Autodesk Fusion 360 part; units mm, degrees
sketch "Sketch1" plane through (0, 0, 0) normal (0, 0, 1) x (1, 0, 0)
  circle A0 centre (0, 0) radius 12.07
  circle A1 centre (0, 0) radius 3.2
  dimension "d1" = 24.14
  dimension "d2" = 6.4
extrude "Extrude1" add sketch "Sketch1" against normal blind 12.4 contours A0 | A1
extrude "Extrude2" add sketch "Sketch1" along normal blind 1 contours A1
sketch "Sketch2" plane through (0, 0, 1) normal (0, 0, 1) x (-1, 0, 0)
  circle A0 centre (0, 0) radius 3.2
  circle A1 centre (0, 0) radius 1
  dimension "d7" = 2
extrude "Extrude3" add sketch "Sketch2" along normal blind 4.7 contours A1
sketch "Sketch3" plane through (0, 0, 0) normal (0, 0, 1) x (1, 0, 0)
  line L0 (0, 0) -> (-8.25, 0) construction
  circle A0 centre (-8.25, 0) radius 0.75
  circle A1 centre (-4.125, -7.1447) radius 0.75
  circle A2 centre (4.125, -7.1447) radius 0.75
  circle A3 centre (8.25, 0) radius 0.75
  circle A4 centre (4.125, 7.1447) radius 0.75
  circle A5 centre (-4.125, 7.1447) radius 0.75
  dimension "d10" = 8.25
  dimension "d11" = 1.5
  dimension "d13" = 360
extrude "Extrude4" cut sketch "Sketch3" against normal blind 2
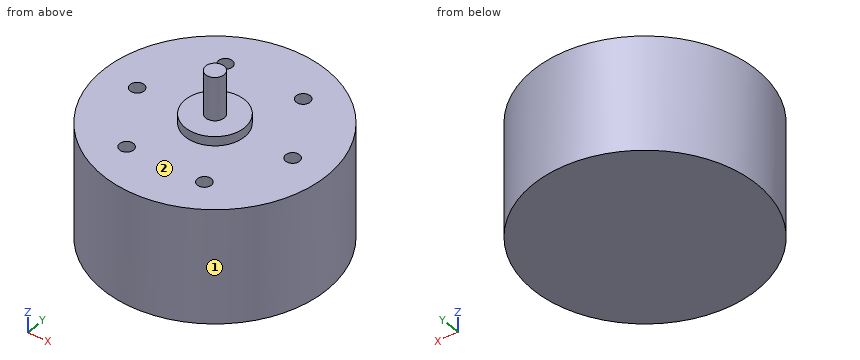
Design review of the part built by this model. Coordinates are the model's own, in mm. Face numbers are marked on the shaded views. A direction names the side the tool comes from. Round coordinates to 2 decimals unless told otherwise and drop trailing zeros. Loops run counter-clockwise (first coordinate to the right, second up) from the corner with the lowest first, then second, coordinate; pieces in that order, holes last. Notation, with made-up numbers: (-21.5, 13) -> (-3.5, 13) arc R10 ccw to (-3.5, 18) -> close; hole circle Ø7 at (-28, 60). An arc over 180 degrees is marked (long way). Use one line per item in the form item = value. Start each with the question number.
Q1. We need section D-D on z = 2.5. Give the boundary of the cut face in (x, y).
Q2. Machinability: for the marked faces 1 and 2, which of the approach directions +Z, -Z, +X, -X, +Y, -Y give a long, thin tool a straight path to every point of the face, cutting with its end or side? Answer none if there is none.
Q3. We need section C-C on z = -1.25. Give the boundary of the cut face in (x, y) (3 decimals).
Q4. We need section B-B on x = 0. Give the boundary of the cut face in (y, z).
Q5. We need section A-A on y = 0. Give the boundary of the cut face in (x, z), then the cut area to 3 significant figures.
Q6. For pin 1 Ø1.5 at (x, z) = (7.5, -5.5) entering from +Y; pin 2 Ø0.9 at (x, y) = (8.25, 0) entering from +Z; pin 3 Ø1.5 at (x, y) = (-8, 7.5) entering from +Z, all flat-tipped, find the tip position at first contact; note any pin that passes through.
Q7. Wall thickness on line 1 along Z through (x, y) = (4.5, 3.25); line 2 along Y through (x, z) = (-8.25, -1.5); line 3 along Y through (x, z) = (3.75, -5): over which ranges is each line inside the solid? List them lowest first. Write a range as [from, to].
Calculated:
q1.outline = circle Ø2 at (0, 0)
q2.face_1 = +Z, -Z
q2.face_2 = +Z
q3.outline = circle Ø24.14 at (0, 0); hole circle Ø1.5 at (-8.25, 0); hole circle Ø1.5 at (-4.125, -7.145); hole circle Ø1.5 at (-4.125, 7.145); hole circle Ø1.5 at (4.125, -7.145); hole circle Ø1.5 at (4.125, 7.145); hole circle Ø1.5 at (8.25, 0)
q4.outline = (-12.07, -12.4) -> (12.07, -12.4) -> (12.07, 0) -> (3.2, 0) -> (3.2, 1) -> (1, 1) -> (1, 5.7) -> (-1, 5.7) -> (-1, 1) -> (-3.2, 1) -> (-3.2, 0) -> (-12.07, 0) -> close
q5.outline = (-12.07, -12.4) -> (12.07, -12.4) -> (12.07, 0) -> (9, 0) -> (9, -2) -> (7.5, -2) -> (7.5, 0) -> (3.2, 0) -> (3.2, 1) -> (1, 1) -> (1, 5.7) -> (-1, 5.7) -> (-1, 1) -> (-3.2, 1) -> (-3.2, 0) -> (-7.5, 0) -> (-7.5, -2) -> (-9, -2) -> (-9, 0) -> (-12.07, 0) -> close
q5.area = 309 mm²
q6.pin_1 = 10.01
q6.pin_2 = -2
q6.pin_3 = 0
q7.line_1 = [-12.4, 0]
q7.line_2 = [-8.81, -0.75], [0.75, 8.81]
q7.line_3 = [-11.47, 11.47]
